Work out the finished part from the listing and answer in its coordinate system (mm). A direction names the side the tool comes from. Round coordinates to 2 decimals unless told otherwise and drop trailing zeros. Write each loop counter-clockwise with the first axis right and the second up, starting at its lowest first coordinate (ties: lowest second). Pieces come first, ordered by that corner, then holes.
from build123d import *

# Parameters (mm, degrees)
SKETCH1_W               = 5
SKETCH1_H               = 47
SKETCH2_W               = 18
SKETCH2_H               = 47
BOSS_EXTRUDE1_DEPTH     = 3.5
SKETCH3_W               = 94
SKETCH3_H               = 94
CUT_EXTRUDE1_DEPTH      = 47
CUT_EXTRUDE1_DEPTH_BACK = 47
SKETCH5_W               = 2
SKETCH5_H               = 53.4
CUT_EXTRUDE2_DEPTH      = 23.5
CUT_EXTRUDE2_DEPTH_BACK = 23.5


with BuildPart() as part:
    # Sketch1 → Revolve1 (revolve)
    with BuildSketch(Plane.XY):
        with Locations((2.5, 0)):
            Rectangle(SKETCH1_W, SKETCH1_H)
    revolve(axis=Axis((0, -23.5, 0), (0, 1, 0)))

    # Sketch2 → Boss-Extrude1 (add)
    with BuildSketch(Plane.XY.offset(-5)):
        with Locations((9, 0)):
            Rectangle(SKETCH2_W, SKETCH2_H)
    extrude(amount=BOSS_EXTRUDE1_DEPTH)

    # Sketch3 → Cut-Extrude1 (cut, two sides)
    with BuildSketch(Plane.XY) as cut_extrude1_sk:
        Rectangle(SKETCH3_W, SKETCH3_H)
        Polygon((-5, 23.5), (-5, 11.75), (5.25, 11.75), (5.25, 0), (-5, 0), (-5, -11.75), (5.25, -11.75), (5.25, -23.5), (18, -23.5), (18, 23.5), align=None, mode=Mode.SUBTRACT)
    extrude(amount=CUT_EXTRUDE1_DEPTH, mode=Mode.SUBTRACT)
    extrude(cut_extrude1_sk.sketch, amount=-CUT_EXTRUDE1_DEPTH_BACK, mode=Mode.SUBTRACT)

    # Sketch4 → Revolve2 (revolve)
    with BuildSketch(Plane.XY):
        Polygon((0, 25.2), (4, 25.2), (4, 24.35), (4.5, 24.35), (4.5, 23.5), (0, 23.5), align=None)
    revolve(axis=Axis((0, 23.5, 0), (0, 1, 0)))

    # Sketch5 → Cut-Revolve1 (revolve, cut)
    with BuildSketch(Plane.XY):
        with Locations((1, 0)):
            Rectangle(SKETCH5_W, SKETCH5_H)
    revolve(axis=Axis((0, -26.7, 0), (0, 1, 0)), mode=Mode.SUBTRACT)

    # Sketch6 → Cut-Revolve2 (revolve, cut)
    with BuildSketch(Plane(origin=(10.5, 0, 0), x_dir=(0, 0, -1), z_dir=(1, 0, 0))):
        Polygon((5, -12.5), (5, -15.25), (4.25, -15.25), (1.5, -18), (1.5, -12.5), align=None)
    revolve(axis=Axis((10.5, -12.5, -1.5), (0, 0, -1)), mode=Mode.SUBTRACT)

    # Sketch7 → Cut-Revolve3 (revolve, cut)
    with BuildSketch(Plane(origin=(10.5, 0, 0), x_dir=(0, 0, -1), z_dir=(1, 0, 0))):
        Polygon((5, 12.5), (5, 9.75), (4.25, 9.75), (1.5, 7), (1.5, 12.5), align=None)
    revolve(axis=Axis((10.5, 12.5, -1.5), (0, 0, -1)), mode=Mode.SUBTRACT)

    # Sketch8 → Cut-Extrude2 (cut, two sides)
    with BuildSketch(Plane(origin=(0, 0, 0), x_dir=(1, 0, 0), z_dir=(0, 1, 0))) as cut_extrude2_sk:
        with BuildLine():
            Line((17, 1.5), (18, 1.5))
            Line((18, 1.5), (18, 2.5))
            ThreePointArc((18, 2.5), (17.707106781, 1.792893219), (17, 1.5))
        make_face()
    extrude(amount=CUT_EXTRUDE2_DEPTH, mode=Mode.SUBTRACT)
    extrude(cut_extrude2_sk.sketch, amount=-CUT_EXTRUDE2_DEPTH_BACK, mode=Mode.SUBTRACT)


solid = part.part
Q1. Find section A-A (y = 12.5). Determine the outline of the cut face in (x, z).
Q2. Find section D-D (z = -1). Determine the outline of the cut face in (x, y).
Q3. Find section B-B (x = 10.5). Determine the outline of the cut face in (y, z).
Q4. Given pin 1 (1.5 mm diameter, centred on y = 15, z = -1.5, fed in from +X); pin 2 (5 mm diameter, centred on y = 19, z = 3, fed in from +X); pin 3 (10 mm diameter, centred on x = 14, y = -0.5, fed in from +Z), each flat-ended and moving along its own axis, determine where each tip first touches the part or whether it passes through.
Q5. The mould has two halves that part along Y. Classify faces 4 (the face through (0.1, -11.75, -2.2)), 5 (the face through (-0.59, 23.92, -4.46)), 6 (the face through (11.55, -15.04, -4.62)): +Y half, -Y half, draft (parallel to the pull), parting line (faces both ways), or undercut.
Q6. Find section C-C (y = -12.5). Determine the outline of the cut face in (x, z).
Q7. A tool of negligible diameter and unlimited length cuts with its end or side. For faces 1 (the face through (5.25, 6, -3)), 2 (the face through (5.25, -18, -3)), 3 (the face through (3, 24.35, 3)), from which of +Z, -Z, +X, -X, +Y, -Y can it reach the whole face along a straight path? Write none if from no direction.
Q8. Find the intervals of material crossed by L1, parallel to Y at x = 10.5, z = -4.55; L2, parallel to Y at x = 2.75, z = 3.5; L3, parallel to Z at x = 0, y = -2.25, in increasing order.
Report:
1. outline: (0, -5) - (7.75, -5) - (7.75, -4.25) - (5, -1.5) - (4.77, -1.5) arc R5 ccw (long way) to start; (13.25, -5) - (18, -5) - (18, -2.5) arc R1 ccw to (17, -1.5) - (16, -1.5) - (13.25, -4.25) - close; hole circle Ø4 at (0, 0)
2. outline: (-4.9, -11.75) - (-1.73, -11.75) - (-1.73, 0) - (-4.9, 0) - close; (-4.9, 11.75) - (-1.73, 11.75) - (-1.73, 25.2) - (-3.87, 25.2) - (-3.87, 24.35) - (-4.39, 24.35) - (-4.39, 23.5) - (-4.9, 23.5) - close; (1.73, -11.75) - (4.9, -11.75) - (4.9, 0) - (1.73, 0) - close; (1.73, 11.75) - (4.9, 11.75) - (4.9, 23.5) - (4.39, 23.5) - (4.39, 24.35) - (3.87, 24.35) - (3.87, 25.2) - (1.73, 25.2) - close
3. outline: (-23.5, -5) - (-15.25, -5) - (-15.25, -4.25) - (-18, -1.5) - (-23.5, -1.5) - close; (-9.75, -5) - (9.75, -5) - (9.75, -4.25) - (7, -1.5) - (-7, -1.5) - (-9.75, -4.25) - close; (15.25, -5) - (23.5, -5) - (23.5, -1.5) - (18, -1.5) - (15.25, -4.25) - close
4. pin 1: stops at x = 17.97
4. pin 2: stops at x = 4.97
4. pin 3: stops at z = -1.5
5. face 4: -Y half
5. face 5: draft
5. face 6: undercut
6. outline: (5.25, -5) - (7.75, -5) - (7.75, -4.25) - (5.25, -1.75) - close; (13.25, -5) - (18, -5) - (18, -2.5) arc R1 ccw to (17, -1.5) - (16, -1.5) - (13.25, -4.25) - close
7. face 1: +Z, -Z, -X
7. face 2: +Z, -Z, -X, -Y
7. face 3: +Y
8. L1: y = -23.5 to -15.25, -9.75 to 9.75, 15.25 to 23.5
8. L2: y = -11.75 to 0, 11.75 to 24.35
8. L3: z = -5 to -2, 2 to 5
